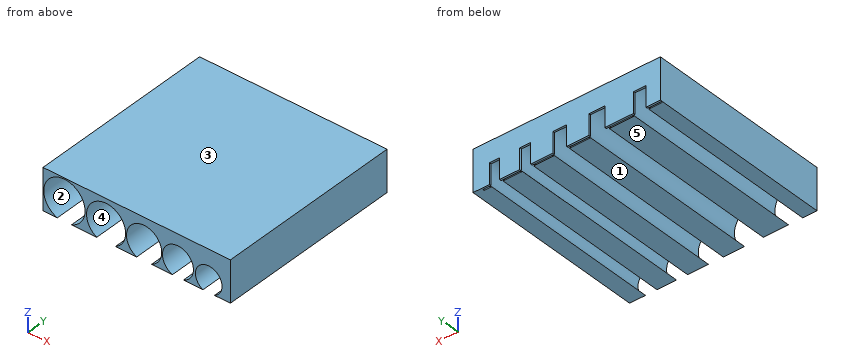
```python
from build123d import *

# Parameters (mm, degrees)
F0_W      = 254
F0_H      = 55.88
F1_DEPTH  = 254
F7_DEPTH  = 251.46
F8_DEPTH  = 251.46
F9_DEPTH  = 251.46
F10_DEPTH = 251.46
F11_DEPTH = 251.46
F12_W     = 18.410387516
F12_H     = 1.8
F12_W_2   = 28.7952162325
F12_W_3   = 28.3505693078
F12_W_4   = 10.2531584787
F13_DEPTH = 28.702
F14_W     = 13.4992599487
F14_H     = 27.94
F14_W_2   = 14.8270688951
F14_W_3   = 18.7435504049
F14_W_4   = 21.5115528554
F14_W_5   = 16.9484987855
F15_DEPTH = 76.2


with BuildPart() as f1:
    # F0 (on Front) → F1 (new body)
    with BuildSketch(Plane.XZ):
        Rectangle(F0_W, F0_H)
    extrude(amount=F1_DEPTH)

    # F6 (on face) → F7 (cut)
    with BuildSketch(Plane.XZ.offset(254)):
        with BuildLine():
            ThreePointArc((105.444855988, -27.94), (97.6680144668, 6.3565803399), (89.8911729455, -27.94))
            Line((89.8911729455, -27.94), (105.444855988, -27.94))
        make_face()
    extrude(amount=-F7_DEPTH, mode=Mode.SUBTRACT)

    # F5 (on face) → F8 (cut)
    with BuildSketch(Plane.XZ.offset(254)):
        with BuildLine():
            ThreePointArc((63.3584037423, -27.94), (55.9246577322, 12.700250005), (48.4909117222, -27.94))
            Line((48.4909117222, -27.94), (63.3584037423, -27.94))
        make_face()
    extrude(amount=-F8_DEPTH, mode=Mode.SUBTRACT)

    # F4 (on face) → F9 (cut)
    with BuildSketch(Plane.XZ.offset(254)):
        with BuildLine():
            ThreePointArc((20.1403424144, -27.94), (10.0701712072, 17.5928532036), (0, -27.94))
            Line((0, -27.94), (20.1403424144, -27.94))
        make_face()
    extrude(amount=-F9_DEPTH, mode=Mode.SUBTRACT)

    # F3 (on face) → F10 (cut)
    with BuildSketch(Plane.XZ.offset(254)):
        with BuildLine():
            ThreePointArc((-28.7952162325, -27.94), (-41.4804015309, 21.8266300514), (-54.1655868292, -27.94))
            Line((-54.1655868292, -27.94), (-28.7952162325, -27.94))
        make_face()
    extrude(amount=-F10_DEPTH, mode=Mode.SUBTRACT)

    # F2 (on face) → F11 (cut)
    with BuildSketch(Plane.XZ.offset(254)):
        with BuildLine():
            Line((-107.5928583741, -27.94), (-88.4136334062, -27.94))
            ThreePointArc((-88.4136334062, -27.94), (-98.0032458901, 26.3666404622), (-107.5928583741, -27.94))
        make_face()
    extrude(amount=-F11_DEPTH, mode=Mode.SUBTRACT)

    # F12 (on face) → F13 (cut)
    with BuildSketch(Plane(origin=(0, 0, -27.94), x_dir=(1, 0, 0), z_dir=(0, 0, -1))):
        with Locations((-116.7980521321, 3.44)):
            Rectangle(F12_W, F12_H)
        Polygon((-70.0032458901, 4.34), (-88.4136334062, 4.34), (-88.4136334062, 2.54), (-70.0032458901, 2.54), (-54.1655868292, 2.54), (-54.1655868292, 4.34), align=None)
        with Locations((-14.3976081163, 3.44)):
            Rectangle(F12_W_2, F12_H)
        with Locations((34.3156270683, 3.44)):
            Rectangle(F12_W_3, F12_H)
        Polygon((89.8911729455, 2.54), (89.8911729455, 4.34), (63.3584037423, 4.34), (63.3584037423, 2.54), (79.6380144668, 2.54), align=None)
        with Locations((110.5714352274, 3.44)):
            Rectangle(F12_W_4, F12_H)
    extrude(amount=-F13_DEPTH, mode=Mode.SUBTRACT)

    # F14 (on face) → F15 (cut)
    with BuildSketch(Plane(origin=(0, 0, 0), x_dir=(-1, 0, 0), z_dir=(0, 1, 0))):
        with Locations((-97.854167223, -13.97)):
            Rectangle(F14_W, F14_H)
        with Locations((-56.2498588115, -13.97)):
            Rectangle(F14_W_2, F14_H)
        with Locations((-9.3717752025, -13.97)):
            Rectangle(F14_W_3, F14_H)
        with Locations((40.9021200612, -13.97)):
            Rectangle(F14_W_4, F14_H)
        with Locations((99.0267731249, -13.97)):
            Rectangle(F14_W_5, F14_H)
    extrude(amount=-F15_DEPTH, mode=Mode.SUBTRACT)


solid = f1.part
```
Design review of the part built by this model. Coordinates are the model's own, in mm. Face numbers are marked on the shaded views. A direction names the side the tool comes from. Give positions to 0.01 mm unless a question says otherwise; leave off trailing zeros. Order: outer loops, then holes, each group sorted by start corner. A loop starts at its lowest first (then second) coordinate and runs counter-clockwise, first axis right, second up. Notation, with made-up numbers: (4, -0.75) -> (44, -0.75) arc R31 cw to (44, 31.25) -> close; hole circle Ø2 at (29.25, -2.75). An arc over 180 degrees is marked (long way). Write item = value, one per line. Start each with the question number.
(1) For the marked faces 4 and 5, list the 3-axis set-ups (+Z, -Z, +X, -X, +Y, -Y) from which the entire face can be reached by the end or side of a thin tool; tool diameter is ignored.
(2) We need section B-B on x = 26. Write out the cut boundary in (y, z).
(3) To check wall thickness, follow line 1 along X through (y, z) = (-108.5, 8); line 2 along X through (y, z) = (-201, -3); line 3 along X through (y, z) = (-173, -1). State the ranges of each line that lie inside material, in increasing order.
(4) We need section D-D on z = -17.5. State how many separate pieces and enclosed holes the cut face has, plus the area to 3 significant figures.
(5) We need section C-C on x = 96. Write out the cut boundary in (y, z).
(6) For pin 1 (1.3 mm diameter, centred on x = 12.5, y = -1, fed in from -Z); pin 2 (2 mm diameter, centred on x = -14, y = -3, fed in from -Z); pin 3 (2 mm diameter, centred on x = -21, z = -2, fed in from -Y); pin 4 (2 mm diameter, centred on x = -34, y = -67, fed in from -Z), all flat-tipped, find the tip position at first contact; note any pin that passes through.
(7) Mouldability with a two-part tool opening along Z and no side actions: class the marked faces 1, 2 and 3 as +Z half, -Z half, draft (parallel to the pull), parting line (faces both ways), or undercut.
(8) We need section A-A on y = -129.5. Write out the cut boundary in (x, z), plus the area to 3 significant figures.
Numbers:
q1.face_4 = -Y
q1.face_5 = -Z, +X, -X, +Y, -Y
q2.outline = (-254, -27.94) -> (-4.34, -27.94) -> (-4.34, -24.08) -> (-254, -24.08) -> close; (-254, 11.5) -> (-2.54, 11.5) -> (-2.54, -27.94) -> (0, -27.94) -> (0, 27.94) -> (-254, 27.94) -> close
q3.line_1 = -127 to -124.29, -71.71 to -64.75, -18.21 to -9.06, 29.2 to 42.68, 69.17 to 127
q3.line_2 = -127 to -125.97, -70.04 to -67.93, -15.03 to -13.58, 33.72 to 35.6, 76.24 to 81.86, 113.47 to 127
q3.line_3 = -127 to -126, -70.01 to -67.72, -15.24 to -13.22, 33.36 to 36.23, 75.62 to 83.14, 112.2 to 127
q4.separate_pieces = 10
q4.enclosed_holes = 0
q4.area = 12,300 mm^2
q5.outline = (-254, 6.28) -> (-2.54, 6.28) -> (-2.54, 0) -> (0, 0) -> (0, 27.94) -> (-254, 27.94) -> close
q6.pin_1 = 0
q6.pin_2 = -27.94
q6.pin_3 = -2.54
q6.pin_4 = 20.43
q7.face_1 = -Z half
q7.face_2 = undercut
q7.face_3 = +Z half
q8.outline = (-127, -27.94) -> (-107.59, -27.94) arc R28 cw (long way) to (-88.41, -27.94) -> (-54.17, -27.94) arc R26.5 cw (long way) to (-28.8, -27.94) -> (0, -27.94) arc R23.88 cw (long way) to (20.14, -27.94) -> (48.49, -27.94) arc R21 cw (long way) to (63.36, -27.94) -> (89.89, -27.94) arc R18.03 cw (long way) to (105.44, -27.94) -> (127, -27.94) -> (127, 27.94) -> (-127, 27.94) -> close
q8.area = 5,470 mm^2
